Input: part model. Units: mm. Frame: model coordinates. A direction names the side the tool comes from. Coordinates: 2 decimals unless noted, no trailing zeros. Loops run counter-clockwise (first coordinate to the right, second up) from the corner with the lowest first, then second, coordinate; pieces in that order, holes last. Notation, with made-up numbers: (37, 87.5) -> (43, 87.5) arc R27 ccw to (43, 117.5) -> close; hole circle Ø1 at (-14.5, -23). An arc over 180 degrees is marked (long way). Answer as a JSON object with one key per item and string values.
from build123d import *

# Parameters (mm, degrees)
BOSS_EXTRUDE1_DEPTH = 12.7
SKETCH2_R           = 3.175
CUT_EXTRUDE1_DEPTH  = 4.175
SKETCH3_R           = 3.175
CUT_EXTRUDE2_DEPTH  = 4.175


with BuildPart() as part:
    # Sketch1 → Boss-Extrude1 (new body)
    with BuildSketch(Plane.XY):
        Polygon((0, 0), (0, 15.875), (3.175, 15.875), (3.175, 3.175), (28.575, 3.175), (28.575, 0), align=None)
    extrude(amount=BOSS_EXTRUDE1_DEPTH)

    # Sketch2 → Cut-Extrude1 (cut, through all)
    with BuildSketch(Plane(origin=(0, 3.175, 0), x_dir=(1, 0, 0), z_dir=(0, 1, 0))):
        with Locations((9.525, -6.35)):
            Circle(SKETCH2_R)
        with Locations((22.225, -6.35)):
            Circle(SKETCH2_R)
    extrude(amount=-CUT_EXTRUDE1_DEPTH, mode=Mode.SUBTRACT)

    # Sketch3 → Cut-Extrude2 (cut, through all)
    with BuildSketch(Plane(origin=(3.175, 0, 0), x_dir=(0, 0, -1), z_dir=(1, 0, 0))):
        with Locations((-6.35, 9.144)):
            Circle(SKETCH3_R)
    extrude(amount=-CUT_EXTRUDE2_DEPTH, mode=Mode.SUBTRACT)


solid = part.part
1. Line query: line 1 along X through (y, z) = (2.2, 6.35) (3 decimals); line 2 along Y through (x, z) = (2.35, 6.35) (3 decimals); line 3 along Y through (x, z) = (13, 11) (3 decimals). Output: solid intervals per line, ascending.
Reply:
{"line 1": "x = 0 to 6.35, 12.7 to 19.05, 25.4 to 28.575", "line 2": "y = 0 to 5.969, 12.319 to 15.875", "line 3": "y = 0 to 3.175"}
2. Section query C-C (x = 21.5). Return loops of the section in (y, z) (3 decimals).
Reply:
{"outline": "(0, 0) -> (3.175, 0) -> (3.175, 3.259) -> (0, 3.259) -> close; (0, 9.441) -> (3.175, 9.441) -> (3.175, 12.7) -> (0, 12.7) -> close"}
3. Section query B-B (y = 2.25). Return loops of the section in (x, z) (3 decimals).
Reply:
{"outline": "(0, 0) -> (28.575, 0) -> (28.575, 12.7) -> (0, 12.7) -> close; hole circle Ø6.35 at (9.525, 6.35); hole circle Ø6.35 at (22.225, 6.35)"}
4. Pin query (flat end, axial travel): P1, Ø7.5, axis at y = 9.144, z = 6.35, coming from the -X side; P2, Ø5, axis at x = 14, z = 3, coming from the +Y side (3 decimals). Return the tip coordinate at first contact, or that it passes through.
Reply:
{"P1": "stops at x = 0", "P2": "stops at y = 3.175"}
5. Section query D-D (y = 9.5). Return loops of the section in (x, z) (3 decimals), plus the area to 3 significant figures.
Reply:
{"outline": "(0, 0) -> (3.175, 0) -> (3.175, 3.195) -> (0, 3.195) -> close; (0, 9.505) -> (3.175, 9.505) -> (3.175, 12.7) -> (0, 12.7) -> close", "area": "20.3 mm2"}
6. Section query A-A (z = 6.35). Return loops of the section in (x, y) (3 decimals), plus the area to 3 significant figures.
Reply:
{"outline": "(0, 0) -> (6.35, 0) -> (6.35, 3.175) -> (3.175, 3.175) -> (3.175, 5.969) -> (0, 5.969) -> close; (0, 12.319) -> (3.175, 12.319) -> (3.175, 15.875) -> (0, 15.875) -> close; (12.7, 0) -> (19.05, 0) -> (19.05, 3.175) -> (12.7, 3.175) -> close; (25.4, 0) -> (28.575, 0) -> (28.575, 3.175) -> (25.4, 3.175) -> close", "area": "70.6 mm2"}
7. Access query for faces 1 (the face through (16, 3.175, 6)), 2 (the face through (2, 15.875, 6)). Directions: +Z, -Z, +X, -X, +Y, -Y. A direction counts if a zero-diameter tool reaches every point of the face in a straight line with its end or side. Return the directions, or none.
Reply:
{"face 1": "+Z, -Z, +X, +Y", "face 2": "+Z, -Z, +X, -X, +Y"}
8. Mould query, pull axis Z, two halves, no side actions, for faces 3 (the face through (10, 3, 0)), 4 (the face through (3.175, 12.4, 7.7)), 5 (the face through (1.61, 6.045, 7.038)). Classes: pulls with the +Z half, pulls with the -Z half, needs draft (parallel to the pull), parting line crosses it, or undercut.
Reply:
{"face 3": "pulls with the -Z half", "face 4": "needs draft", "face 5": "undercut"}
